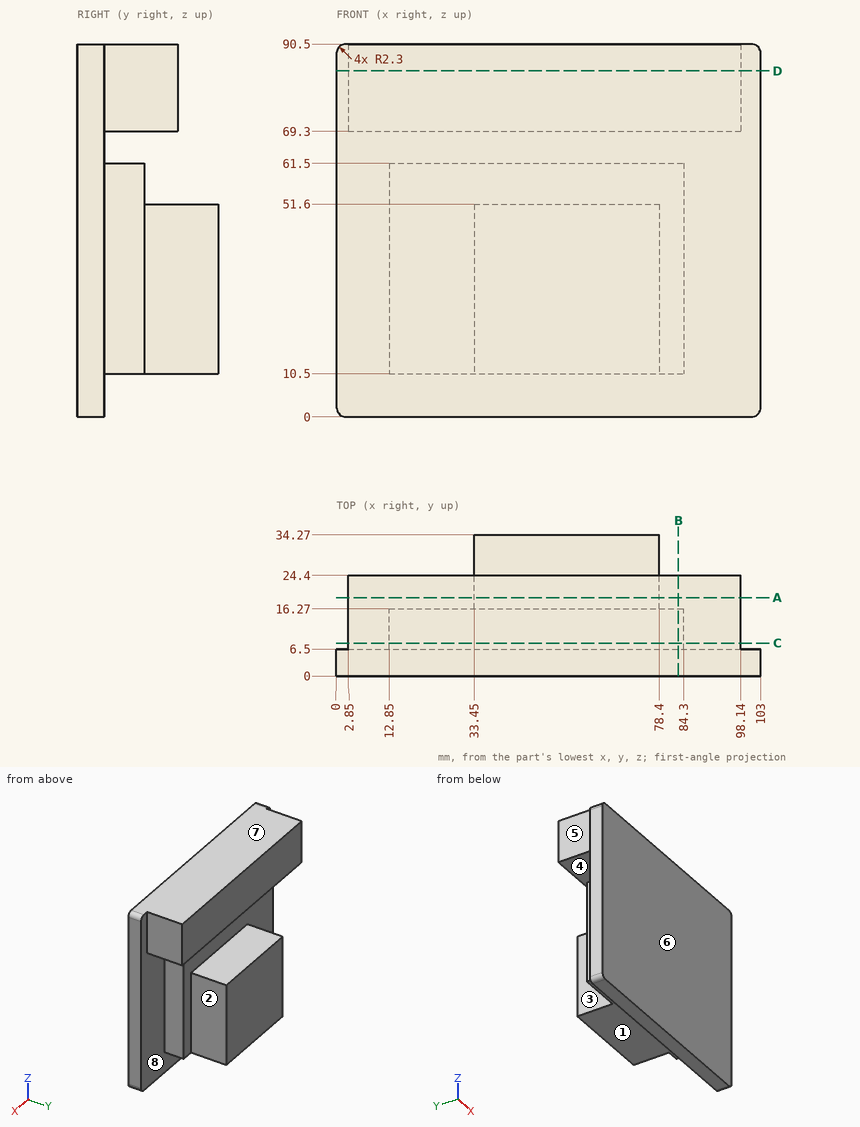
Job drawing, mm, ordinate dimensions from the low corner. One solid piece. A direction names the side the tool comes from. Give positions to 0.01 mm unless a question says otherwise; leave off trailing zeros. Loops run counter-clockwise (first coordinate to the right, second up) from the corner with the lowest first, then second, coordinate; pieces in that order, holes last. Notation, with made-up numbers: M 84.25,-34.5 L 140.25,-34.5 A15 cw 140.25,-16.5 Z; hole C -12.75,12 d10. An arc over 180 degrees is marked long. Put each result on its own line as item: value. Start each with the question number.
1) Saw through at A-A (y = 19). List the corners of the cut face in (x, z).
2) Probe probe 1 along Z at (x, y) = (49, 10); probe 2 along Z at (x, y) = (31, 20); probe 3 along Y at (x, z) = (32.5, 15). List the from-to ranges inside material, lowest first.
3) Pull direction Z, two halves, no side cores. Call the marked faces 6, 7 and 8: +Z half, -Z half, draft (parallel to the pull), parting line (faces both ways), or undercut.
4) Flat gauge pins, fed straight in: pin 1 (20 mm diameter, centred on y = 21, z = 38, fed in from -X); pin 2 (10 mm diameter, centred on x = 42, z = 76, fed in from +Y); pin 3 (5 mm diameter, centred on x = 53, y = 14, fed in from -Z); pin 4 (19.5 mm diameter, centred on y = 14.5, z = 79.5, fed in from +X). Where does each tip first touch, or does it go through?
5) Saw through at C-C (y = 8). List the corners of the cut face in (x, z).
6) Saw through at D-D (z = 84). List the corners of the cut face in (x, y).
7) 3-axis set-ups, long thin cutter, end or side, ignore diameter. For the marked faces 1, 2, 3, 4 and 5: which of +Z, -Z, +X, -X, +Y, -Y reach the whole face in a straight line?
8) Saw through at B-B (x = 83). List the corners of the cut face in (y, z).
Numbers:
1. outline: M 2.85,69.3 L 98.14,69.3 L 98.14,90.5 L 2.85,90.5 Z; M 33.45,10.5 L 78.4,10.5 L 78.4,51.6 L 33.45,51.6 Z
2. probe 1: 10.5 to 61.5, 69.3 to 90.5
2. probe 2: 69.3 to 90.5
2. probe 3: 0 to 16.27
3. face 6: draft
3. face 7: +Z half
3. face 8: undercut
4. pin 1: x = 12.85
4. pin 2: y = 24.4
4. pin 3: z = 10.5
4. pin 4: x = 103
5. outline: M 2.85,69.3 L 98.14,69.3 L 98.14,90.5 L 2.85,90.5 Z; M 12.85,10.5 L 84.3,10.5 L 84.3,61.5 L 12.85,61.5 Z
6. outline: M 0,0 L 103,0 L 103,6.5 L 98.14,6.5 L 98.14,24.4 L 2.85,24.4 L 2.85,6.5 L 0,6.5 Z
7. face 1: -Z, +X, -X, +Y
7. face 2: -Z, +X, +Y
7. face 3: -Z, -X, +Y
7. face 4: +X, -X, +Y
7. face 5: +Z, -Z, -X, +Y
8. outline: M 0,0 L 6.5,0 L 6.5,10.5 L 16.27,10.5 L 16.27,61.5 L 6.5,61.5 L 6.5,69.3 L 24.4,69.3 L 24.4,90.5 L 0,90.5 Z
